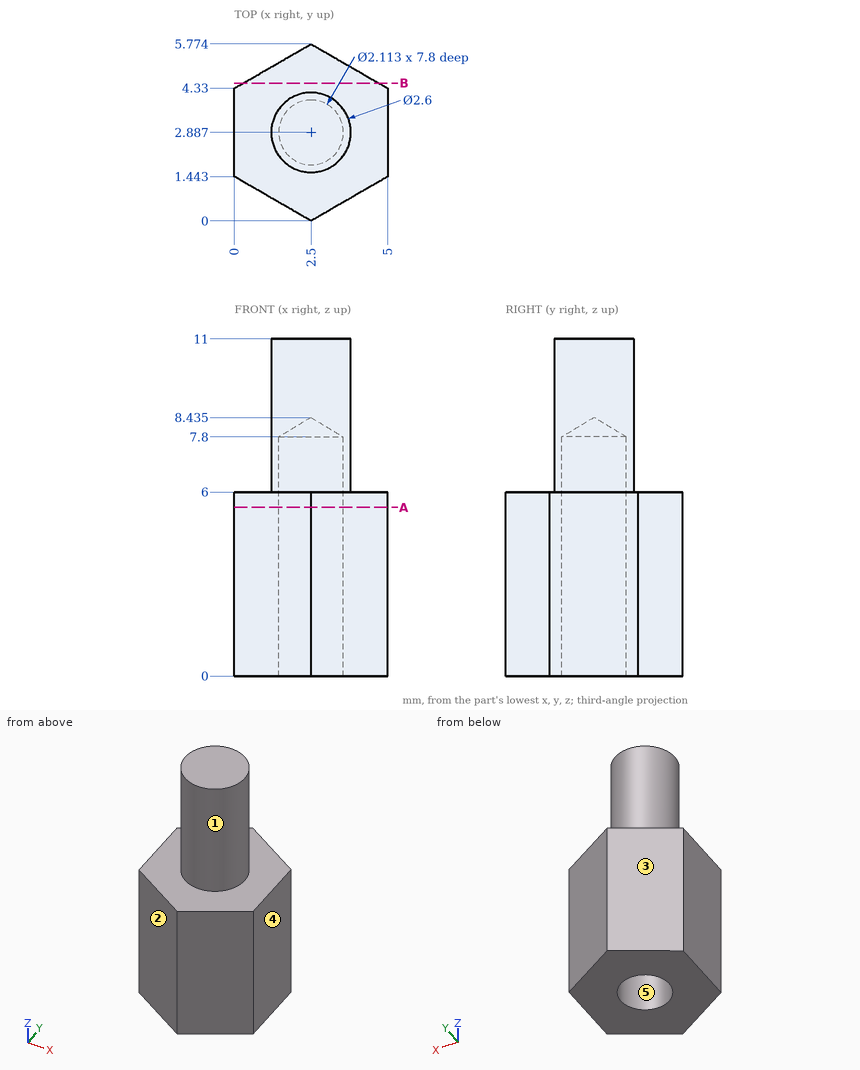
Input: dimensioned drawing with shaded views. Units: mm. Origin: part minimum x, y, z. A direction names the side the tool comes from. Round coordinates to 2 decimals unless told otherwise and drop trailing zeros. Loops run counter-clockwise (first coordinate to the right, second up) from the corner with the lowest first, then second, coordinate; pieces in that order, holes last. Notation, with made-up numbers: (15, 24.25) -> (52, 24.25) arc R18 cw to (52, 39.25) -> close; hole circle Ø7 at (71, -13.75). An arc over 180 degrees is marked (long way). Use one line per item in the form item = value. Start each with the question number.
1) Access query for the marked faces 1 and 2. Directions: +Z, -Z, +X, -X, +Y, -Y. A direction counts if a zero-diameter tool reaches every point of the face in a straight line with its end or side. Return the directions, or none.
2) Section A-A on z = 5.5. Output: boundary loops of the cut face in (x, y).
3) Section B-B on y = 4.5. Output: boundary loops of the cut face in (x, z), then the cut area to 3 significant figures.
4) First-contact query: P1, Ø2, axis at x = 1, z = 8.5, coming from the +Y side; P2, Ø3, axis at y = 3, z = 10, coming from the -X side; P3, Ø1, axis at x = 2, z = 10, coming from the +Y side. Flat tips, straight axial feed; report the tip coordinate or a pass-through.
5) Line query: L1, parallel to X at y = 2.95, z = 1 (1 decimal); L2, parallel to Z at x = 0.6, y = 2.1; L3, parallel to X at y = 2.1, z = 2.5 (1 decimal). Output: solid intervals per line, ascending.
6) Draft query along Y for the marked faces 3, 4 and 5. Return one class per face: released by +Y, released by -Y, zero draft, split by the parting line, or undercut.
Response:
q1.face_1 = +Z
q1.face_2 = +Z, -Z, -X, -Y
q2.outline = (0, 1.44) -> (2.5, 0) -> (5, 1.44) -> (5, 4.33) -> (2.5, 5.77) -> (0, 4.33) -> close; hole circle Ø2.11 at (2.5, 2.89)
q3.outline = (0.29, 0) -> (4.71, 0) -> (4.71, 6) -> (0.29, 6) -> close
q3.area = 26.5 mm^2
q4.P1 = 4.09
q4.P2 = 1.2
q4.P3 = 4.19
q5.L1 = 0 to 1.4, 3.6 to 5
q5.L2 = 0 to 6
q5.L3 = 0 to 1.8, 3.2 to 5
q6.face_3 = released by +Y
q6.face_4 = zero draft
q6.face_5 = undercut
